Read the model definition and answer for the solid it produces. Units are mm, in the model's axes. A direction names the side the tool comes from. Give positions to 0.01 mm unless a question says otherwise; leave off trailing zeros. Loops run counter-clockwise (first coordinate to the right, second up) from the corner with the lowest first, then second, coordinate; pieces in that order, holes last. Notation, with made-up numbers: (61.25, 23) - (115.25, 23) arc R29 ccw to (115.25, 43) - close; hole circle Ø6 at (78.25, 60). An arc over 180 degrees is marked (long way). Put each result on its own line as item: value. Start each with the question number.
1. Consider L1, parallel to Y at x = 12, z = 57; L2, parallel to Z at x = 122, y = -37. Determine where each line is inside the solid, lowest interval first. Write a range as from..to.
2. A cutting plane is placed at A-A, the plane x = 152.4. Determine the outline of the cut face in (y, z).
3. Given pin 1 Ø1.5 at (x, y) = (91, -53) entering from -Z; pin 2 Ø1 at (x, y) = (142.5, -10.5) entering from +Z; pin 3 Ø1 at (y, z) = (-25.5, 17.5) entering from +X, each flat-ended and moving along its own axis, determine where each tip first touches the part or whether it passes through.
4. A cutting plane is placed at D-D, the plane z = 26. Determine the outline of the cut face in (x, y).
5. For faces 1 (the flat face through (25.4, -41, 36)), 2 (the cylindrical face through (172.084, -35.076, 6.439)), determine the directions among +Z, -Z, +X, -X, +Y, -Y from which every point of the face is accessible in a straight line to the end or side of a thin tool.
6. A cutting plane is placed at B-B, the plane z = 40.5. Determine the outline of the cut face in (x, y).
7. A cutting plane is placed at C-C, the plane y = -24.5. Determine the outline of the cut face in (x, z), plus the area to 3 significant figures.
8. For a pull along Y with two mould halves and no side action, classify faces 3 (the flat face through (67, -82.55, 12)), 4 (the cylindrical face through (12.878, -43.962, 77.612)), 5 (the flat face through (109, -41, 12.7)) as released by +Y, released by -Y, zero draft, split by the parting line, or undercut.
```python
from build123d import *

# Parameters (mm, degrees)
F1_DEPTH = 82.55
F3_DEPTH = 25.4
F4_R     = 20.6375
F5_DEPTH = 25.4
F6_R     = 20.6375
F7_DEPTH = 25.4


with BuildPart() as f1:
    # F0 (on Front) → F1 (new body)
    with BuildSketch(Plane.XZ):
        Polygon((0, 114.3), (0, 0), (190.5, 0), (190.5, 12.7), (25.4, 12.7), (25.4, 114.3), align=None)
    extrude(amount=F1_DEPTH)

    # F2 (on face) → F3 (cut)
    with BuildSketch(Plane.YZ.offset(25.4)):
        with BuildLine():
            ThreePointArc((-82.55, 57.15), (-41.275, 98.425), (0, 57.15))
            Line((0, 57.15), (0, 114.3))
            Line((0, 114.3), (-82.55, 114.3))
            Line((-82.55, 114.3), (-82.55, 57.15))
        make_face()
    extrude(amount=-F3_DEPTH, mode=Mode.SUBTRACT)

    # F4 (on face) → F5 (cut, through all)
    with BuildSketch(Plane.YZ.offset(25.4)):
        with Locations((-41.275, 57.15)):
            Circle(F4_R)
    extrude(amount=-F5_DEPTH, mode=Mode.SUBTRACT)

    # F6 (on face) → F7 (cut)
    with BuildSketch(Plane.XY.offset(12.7)):
        with Locations((76.2, -41.275)):
            Circle(F6_R)
        with Locations((152.4, -41.275)):
            Circle(F6_R)
    extrude(amount=-F7_DEPTH, mode=Mode.SUBTRACT)


solid = f1.part
```
Return value:
1. L1: y = -82.55..-61.91, -20.64..0
1. L2: z = 0..12.7
2. outline: (-82.55, 0) - (-61.91, 0) - (-61.91, 12.7) - (-82.55, 12.7) - close; (-20.64, 0) - (0, 0) - (0, 12.7) - (-20.64, 12.7) - close
3. pin 1: passes through
3. pin 2: stops at z = 12.7
3. pin 3: stops at x = 25.4
4. outline: (0, -82.55) - (25.4, -82.55) - (25.4, 0) - (0, 0) - close
5. face 1: +Z, +X, +Y, -Y
5. face 2: +Z, -Z
6. outline: (0, -82.55) - (25.4, -82.55) - (25.4, -53.47) - (0, -53.47) - close; (0, -29.08) - (25.4, -29.08) - (25.4, 0) - (0, 0) - close
7. outline: (0, 0) - (64.18, 0) - (64.18, 12.7) - (25.4, 12.7) - (25.4, 45.13) - (0, 45.13) - close; (0, 69.17) - (25.4, 69.17) - (25.4, 94.86) - (0, 94.86) - close; (88.22, 0) - (140.38, 0) - (140.38, 12.7) - (88.22, 12.7) - close; (164.42, 0) - (190.5, 0) - (190.5, 12.7) - (164.42, 12.7) - close
7. area: 3,280 mm2
8. face 3: released by -Y
8. face 4: undercut
8. face 5: zero draft
